Autodesk Inventor part; units mm, degrees
ref_plane "YZ Plane" through (0, 0, 0) normal (1, 0, 0) x (0, 1, 0)
ref_plane "XZ Plane" through (0, 0, 0) normal (0, 1, 0) x (-1, 0, 0)
ref_plane "XY Plane" through (0, 0, 0) normal (0, 0, 1) x (1, 0, 0)
sketch "Sketch1" plane through (0, 0, 0) normal (0, 1, 0) x (-1, 0, 0)
  circle A0 centre (0, 0) radius 24.5
  dimension "d0" = 49
extrude "Extrusion1" add sketch "Sketch1" along normal blind 9
sketch "Sketch2" plane through (0, 0, 0) normal (0, -1, 0) x (1, 0, 0)
  point P0 (0, 0)
sketch "Sketch3" plane through (0, 0, 0) normal (0, -1, 0) x (1, 0, 0)
  circle A0 centre (0, 0) radius 18
  dimension "d3" = 36
extrude "Extrusion2" cut sketch "Sketch3" against normal blind 2
chamfer "Chamfer1" distance 2 angle 45 1 edges at (-18, 2, 0)
hole "Hole1" at (0, 0, 0) direction (0, 1, 0) diameter 8 end through all
sketch "Sketch4" plane through (0, 2, 0) normal (0, -1, 0) x (1, 0, 0)
  circle A0 centre (-12, 0) radius 3.5
  point P0 (0, 0)
  dimension "d17" = 7
  dimension "d18" = 12
extrude "Extrusion3" cut sketch "Sketch4" against normal through all
pattern_circular "Circular Pattern1" count 4 over 360 about axis through (0, -10, 0) along (0, 1, 0) of "Extrusion3"
chamfer "Chamfer2" distance 1 angle 45 2 edges at (24.5, 0, 0) (24.5, 9, 0)
properties part number "Wheel" material "Iron, Gray"
Verification items for the finished model (mm, model axes). A direction names the side the tool comes from. Give positions to 0.01 mm unless a question says otherwise; leave off trailing zeros. Loops run counter-clockwise (first coordinate to the right, second up) from the corner with the lowest first, then second, coordinate; pieces in that order, holes last. Notation, with made-up numbers: (52.5, 72) - (99.5, 72) arc R8 ccw to (99.5, 85) - close; hole circle Ø2 at (-2, -9.75). An arc over 180 degrees is marked (long way). Write item = value, one per line. Start each with the question number.
Q1. Cross-section at C-C, the plane y = 3.75. Enter the section's corners in (x, z), and give its area (3 significant figures).
Q2. Mould release check, pull along Z, two halves, no side actions. Record for faces 3 (the face through (-3.496, 1.875, -15.742)), 4 (the face through (-13.17, 4.45, -20.66)), 5 (the face through (0, 9, -5)): released by +Z, released by -Z, zero draft, split by the parting line, or undercut.
Q3. Tool access check on faces 1 (the face through (3, 2, -3)), 2 (the face through (3.905, 5.549, 0.867)). Record the directions out of +Z, -Z, +X, -X, +Y, -Y that give a thin tool (end or side, any length) a straight path to the whole face; none if there is none.
Q4. Thickness scan on line 1 (Z direction, x = 0.5, y = 2.75); line 2 (Y direction, x = 9, z = 6.5); line 3 (Y direction, x = -7, z = -15.5). Record the ranges inside material, lowest first.
Q5. Depth check by flat-ended pin: P1, Ø4, axis at x = 0, z = -12, coming from the -Y side; P2, Ø1.5, axis at y = 3.5, z = 12, coming from the +X side; P3, Ø1.5, axis at y = 5.5, z = -6, coming from the -X side; P4, Ø1.5, axis at y = 7.5, z = 17.5, coming from the -X side. Enter the tip coordinate at first touch or a pass-through.
Q6. Cross-section at A-A, the plane x = 0. State how many separate pieces and enclosed holes the cut face has, and give its area (3 significant figures).
Answer key:
q1.outline = circle Ø49 at (0, 0); hole circle Ø7 at (-12, 0); hole circle Ø8 at (0, 0); hole circle Ø7 at (0, -12); hole circle Ø7 at (0, 12); hole circle Ø7 at (12, 0)
q1.area = 1,680 mm^2
q2.face_3 = undercut
q2.face_4 = split by the parting line
q2.face_5 = zero draft
q3.face_1 = -Y
q3.face_2 = +Y, -Y
q4.line_1 = -24.49 to -15.46, -8.54 to -3.97, 3.97 to 8.54, 15.46 to 24.49
q4.line_2 = 2 to 9
q4.line_3 = 0.99 to 9
q5.P1 = through
q5.P2 = 21.76
q5.P3 = -23.93
q5.P4 = -17.88
q6.separate_pieces = 4
q6.enclosed_holes = 0
q6.area = 217 mm^2
